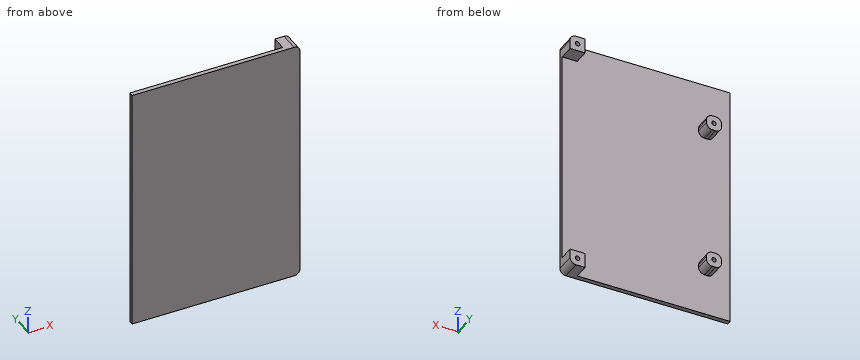
Autodesk Inventor part; units mm, degrees
ref_plane "YZ Plane" through (0, 0, 0) normal (1, 0, 0) x (0, 1, 0)
ref_plane "XZ Plane" through (0, 0, 0) normal (0, 1, 0) x (-1, 0, 0)
ref_plane "XY Plane" through (0, 0, 0) normal (0, 0, 1) x (1, 0, 0)
sketch "Эскиз1" plane through (0, 0, 0) normal (0, 1, 0) x (-1, 0, 0)
  line L0 (0, 0) -> (56, 0)
  line L1 (56, 0) -> (56, -82)
  line L2 (56, -82) -> (0, -82)
  line L3 (0, -82) -> (0, 0)
  dimension "d0" = 56
  dimension "d1" = 82
extrude "Выдавливание1" add sketch "Эскиз1" along normal blind 1.5
sketch "Эскиз2" plane through (0, 1.5, 0) normal (0, 1, 0) x (1, 0, 0)
  line L0 (-56, 0) -> (0, 0)
  line L1 (0, 0) -> (-5, 0)
  line L2 (-5, 0) -> (-5, 5)
  line L3 (-5, 5) -> (0, 5)
  line L4 (0, 5) -> (0, 0)
  line L5 (0, 0) -> (0, 82)
  line L6 (0, 82) -> (-5, 82)
  line L7 (-5, 82) -> (-5, 77)
  line L8 (-5, 77) -> (0, 77)
  line L9 (0, 77) -> (0, 82)
  line L10 (-50.5, 14) -> (-45.5, 14)
  line L11 (-45.5, 14) -> (-45.5, 19)
  line L12 (-45.5, 19) -> (-50.5, 19)
  line L13 (-50.5, 19) -> (-50.5, 14)
  line L14 (-50.5, 63) -> (-45.5, 63)
  line L15 (-45.5, 63) -> (-45.5, 68)
  line L16 (-45.5, 68) -> (-50.5, 68)
  line L17 (-50.5, 68) -> (-50.5, 63)
  line L18 (-56, 82) -> (-56, 0)
  line L19 (0, 82) -> (-56, 82)
  dimension "d4" = 5
  dimension "d5" = 5
  dimension "d6" = 5
  dimension "d7" = 5
  dimension "d8" = 5
  dimension "d9" = 5
  dimension "d10" = 5
  dimension "d11" = 5
  dimension "d12" = 14
  dimension "d13" = 5.5
  dimension "d14" = 14
extrude "Выдавливание2" add sketch "Эскиз2" along normal blind 5 contours L2 L3 L4 L0 | L6 L5 L8 L7 | L13 L12 L11 L10 | L17 L16 L15 L14
sketch "Эскиз3" plane through (0, 6.5, 0) normal (0, 1, 0) x (1, 0, 0)
  circle A0 centre (-2.5, 2.5) radius 0.75
  line L0 (-5, 0) -> (0, 0)
  line L1 (0, 0) -> (0, 5)
  circle A1 centre (-2.5, 79.5) radius 0.75
  line L2 (0, 77) -> (0, 82)
  line L3 (0, 82) -> (-5, 82)
  circle A2 centre (-48, 16.5) radius 0.75
  line L4 (-56, 0) -> (-5, 0)
  circle A3 centre (-48, 65.5) radius 0.75
  line L5 (-5, 82) -> (-56, 82)
  line L6 (-45.5, 14) -> (-45.5, 19)
  line L7 (-45.5, 63) -> (-45.5, 68)
  dimension "d17" = 1.5
  dimension "d18" = 2.5
  dimension "d19" = 2.5
  dimension "d20" = 1.5
  dimension "d21" = 2.5
  dimension "d22" = 2.5
  dimension "d23" = 1.5
  dimension "d24" = 16.5
  dimension "d25" = 1.5
  dimension "d26" = 16.5
  dimension "d27" = 2.5
  dimension "d28" = 2.5
extrude "Выдавливание3" cut sketch "Эскиз3" against normal blind 5
fillet "Сопряжение1" radius 2 10 edges at (0, 3.25, 0) (0, 3.25, -82) (-45.5, 4, -14) (-45.5, 4, -19) (-50.5, 4, -14) (-50.5, 4, -19) (-45.5, 4, -63) (-45.5, 4, -68) (-50.5, 4, -68) (-50.5, 4, -63)
properties part number "VIM1_Holder"
Design review of the part built by this model. Coordinates are the model's own, in mm. Give positions to 0.01 mm unless a question says otherwise; leave off trailing zeros. Write each loop counter-clockwise with the first axis right and the second up, starting at its lowest first coordinate (ties: lowest second). Pieces come first, ordered by that corner, then holes. Notation, with made-up numbers: (-8, -31.75) -> (31, -31.75) arc R19 cw to (31, -12.75) -> close; hole circle Ø4 at (-26.75, 83.25). An arc over 180 degrees is marked (long way). Answer in a Markdown table with one row per item.
(1) Consider section B-B (z = -73). State the section outline as (x, y) points, then the cut area to 3 significant figures.
Results:
| item | result |
|---|---|
| outline | (-56, 0) -> (0, 0) -> (0, 1.5) -> (-56, 1.5) -> close |
| area | 84.0 mm2 |
(2) Consider section C-C (x = -34.5). State the section outline as (y, z) points, then the cut area to 3 significant figures.
Results:
| item | result |
|---|---|
| outline | (0, -82) -> (1.5, -82) -> (1.5, 0) -> (0, 0) -> close |
| area | 123 mm2 |
(3) To check wall thickness, follow probe 1 along Z at (x, y) = (-48, 3.7); probe 2 along X at (y, z) = (4.1, -65.5); probe 3 along X at (y, z) = (5.3, -79.5). State the ranges of each line that lie inside material, in increasing order.
Results:
| item | result |
|---|---|
| probe 1 | -68 to -66.25, -64.75 to -63, -19 to -17.25, -15.75 to -14 |
| probe 2 | -50.5 to -48.75, -47.25 to -45.5 |
| probe 3 | -5 to -3.25, -1.75 to 0 |
(4) Consider section A-A (y = 5.5). Count the separate pieces of the cut face and the enclosed holes in it, then the cut area to 3 significant figures.
Results:
| item | result |
|---|---|
| separate pieces | 4 |
| enclosed holes | 4 |
| area | 84.3 mm2 |
(5) Clearance check with flat-ended pins moving along their axes: pin 1 (0.5 mm diameter, centred on y = 3.5, z = -16.5, fed in from +X); pin 2 (1 mm diameter, centred on x = -41.5, z = -44.5, fed in from +Y); pin 3 (0.5 mm diameter, centred on x = -48, y = 3, fed in from -Z). State where each tip first meets the part, or that it passes through.
Results:
| item | result |
|---|---|
| pin 1 | x = -45.5 |
| pin 2 | y = 1.5 |
| pin 3 | z = -68 |
